Autodesk Inventor part; units mm, degrees
ref_plane "YZ Plane" through (0, 0, 0) normal (1, 0, 0) x (0, 1, 0)
ref_plane "XZ Plane" through (0, 0, 0) normal (0, 1, 0) x (-1, 0, 0)
ref_plane "XY Plane" through (0, 0, 0) normal (0, 0, 1) x (1, 0, 0)
sketch "Sketch1" plane through (0, 0, 0) normal (1, 0, 0) x (0, 1, 0)
  line L0 (0, 0) -> (0, 5)
  line L1 (0, 5) -> (-3, 5)
  line L2 (-3, 5) -> (-3, 8)
  line L3 (-3, 8) -> (0, 8)
  line L4 (0, 8) -> (0, 11)
  line L5 (0, 11) -> (2.1716, 11)
  line L6 (11, 0) -> (8, 0)
  line L7 (8, 0) -> (8, -3)
  line L8 (8, -3) -> (5, -3)
  line L9 (5, -3) -> (5, 0)
  line L10 (5, 0) -> (0, 0)
  line L11 (11, 0) -> (11, 2.1716)
  line L12 (10.4142, 3.5858) -> (3.5858, 10.4142)
  arc A0 (3.5858, 10.4142) -> (2.1716, 11) centre (2.1716, 9) ccw
  arc A1 (11, 2.1716) -> (10.4142, 3.5858) centre (9, 2.1716) ccw
  point P0 (3, 11)
  point P1 (11, 3)
  dimension "d0" = 5
  dimension "d1" = 3
  dimension "d2" = 3
  dimension "d3" = 5
  dimension "d4" = 3
  dimension "d5" = 3
  dimension "d6" = 3
  dimension "d7" = 3
  dimension "d8" = 3
  dimension "d9" = 3
  dimension "d10" = 3
  dimension "d11" = 3
  dimension "d14" = 2
extrude "Extrusion1" add sketch "Sketch1" along normal blind 3
properties part number "Endplate_B Support"
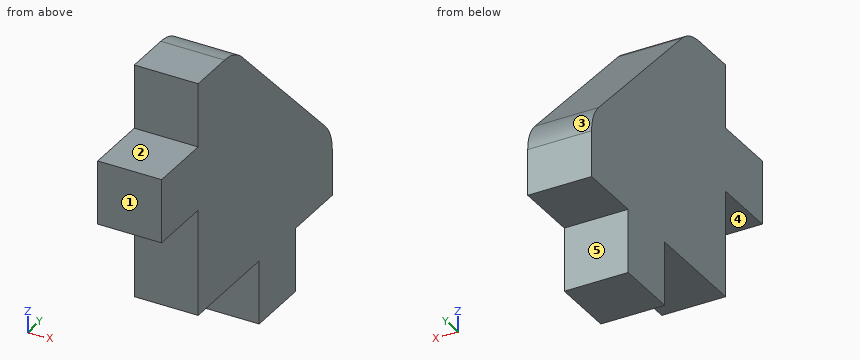
Work out the finished part from the listing and answer in its coordinate system (mm). Face numbers are marked on the shaded views. A direction names the side the tool comes from. Give positions to 0.01 mm unless a question says otherwise; leave off trailing zeros. Write each loop counter-clockwise with the first axis right and the second up, starting at its lowest first coordinate (ties: lowest second). Pieces come first, ordered by that corner, then holes. Notation, with made-up numbers: (42, -31.5) -> (49, -31.5) arc R25 cw to (49, 3.5) -> close; hole circle Ø3 at (75, 72). An arc over 180 degrees is marked (long way). Write item = value, one per line.
Q1. Section A-A on x = 1.35 is taken. Determine the outline of the cut face in (y, z).
Computed values:
outline = (-3, 5) -> (0, 5) -> (0, 0) -> (5, 0) -> (5, -3) -> (8, -3) -> (8, 0) -> (11, 0) -> (11, 2.17) arc R2 ccw to (10.41, 3.59) -> (3.59, 10.41) arc R2 ccw to (2.17, 11) -> (0, 11) -> (0, 8) -> (-3, 8) -> close
Q2. Section C-C on z = -1 is taken. Determine the outline of the cut face in (x, y), and give its area (3 significant figures).
Computed values:
outline = (0, 5) -> (3, 5) -> (3, 8) -> (0, 8) -> close
area = 9.00 mm^2
Q3. Flat-ended cylindrical pins translate along their axes: pin 1 Ø0.9 at (x, z) = (2, -1) entering from -Y; pin 2 Ø0.9 at (x, y) = (2, 9.5) entering from -Z; pin 3 Ø1.5 at (x, z) = (1.5, -2) entering from +Y. Find the tip coordinate at first contact, or state that the pin passes through.
Computed values:
pin_1 = 5
pin_2 = 0
pin_3 = 8
Q4. A tool of negligible diameter and unlimited length cuts with its end or side. For the marked faces 1, 2, 3, 4 and 5, from which of +Z, -Z, +X, -X, +Y, -Y can it reach the whole face along a straight path? Write none if from no direction.
Computed values:
face_1 = +Z, -Z, +X, -X, -Y
face_2 = +Z, +X, -X, -Y
face_3 = +Z, +X, -X, +Y
face_4 = -Z, +X, -X, -Y
face_5 = -Z, +X, -X, +Y
Q5. Section B-B on y = 8.5 is taken. Determine the outline of the cut face in (x, z), and give its area (3 significant figures).
Computed values:
outline = (0, 0) -> (3, 0) -> (3, 5.5) -> (0, 5.5) -> close
area = 16.5 mm^2
Q6. Consider line 1 along Z through (x, y) = (2.55, 0.5); line 2 along Y through (x, z) = (2.3, -0.25). Determine where each line is inside the solid, lowest interval first.
Computed values:
line_1 = 0 to 11
line_2 = 5 to 8
